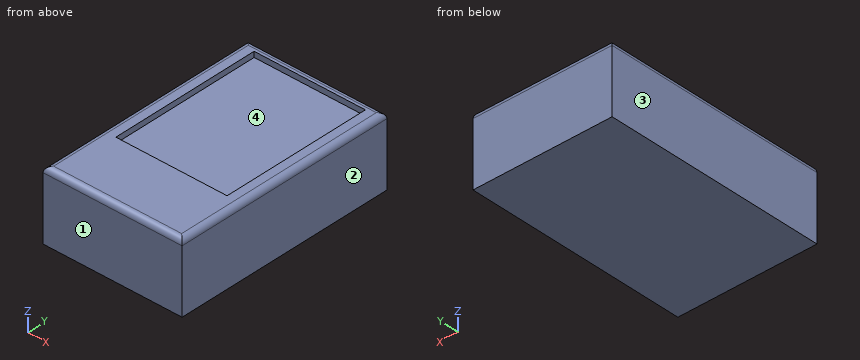
from build123d import *

# Parameters (mm, degrees)
F0_W     = 63.5
F0_H     = 101.6
F1_DEPTH = 31.75
F2_R     = 2.54
F3_W     = 50.8
F3_H     = 68.58
F4_DEPTH = 2.54


with BuildPart() as f1:
    # F0 (on Top) → F1 (new body)
    with BuildSketch(Plane.XY):
        Rectangle(F0_W, F0_H)
    extrude(amount=F1_DEPTH)

    # F2
    f2_edges = [f1.edges().sort_by_distance(p)[0] for p in [
        (0, 50.8, 31.75),
        (-31.75, 0, 31.75),
        (31.75, 0, 31.75),
        (0, -50.8, 31.75),
    ]]
    fillet(f2_edges, radius=F2_R)

    # F3 (on face) → F4 (cut)
    with BuildSketch(Plane.XY.offset(31.75)):
        with Locations((0, 12.7)):
            Rectangle(F3_W, F3_H)
    extrude(amount=-F4_DEPTH, mode=Mode.SUBTRACT)


solid = f1.part
Verification items for the finished model (mm, model axes). Face numbers are marked on the shaded views. Round coordinates to 2 decimals unless told otherwise and drop trailing zeros. Loops run counter-clockwise (first coordinate to the right, second up) from the corner with the lowest first, then second, coordinate; pieces in that order, holes last. Notation, with made-up numbers: M 55,23.25 L 98,23.25 A9 ccw 98,35.25 Z; hole C -19,-24.5 d10. An arc over 180 degrees is marked long. Write each question's results on one line, items separated by ' | '.
1) Section check B-B on y = 11. Record the boundary of the cut face in (x, z).
Checks:
outline: M -31.75,0 L 31.75,0 L 31.75,29.21 A2.54 ccw 29.21,31.75 L 25.4,31.75 L 25.4,29.21 L -25.4,29.21 L -25.4,31.75 L -29.21,31.75 A2.54 ccw -31.75,29.21 Z
2) Gauge pin test, flat ends, axial feed: P1, Ø2, axis at x = 9, z = 30.5, coming from the +Y side; P2, Ø0.8, axis at y = 0, z = 31, coming from the -X side; P3, Ø6, axis at x = -0.5, y = -18, coming from the +Z side. Record the tip position at first contact, or that the pin passes through.
Checks:
P1: stops at y = 50.78 | P2: stops at x = -31.34 | P3: stops at z = 29.21
3) Section check A-A on x = -3.5. Record the boundary of the cut face in (y, z), then the cut area to 3 significant figures.
Checks:
outline: M -50.8,0 L 50.8,0 L 50.8,29.21 A2.54 ccw 48.26,31.75 L 46.99,31.75 L 46.99,29.21 L -21.59,29.21 L -21.59,31.75 L -48.26,31.75 A2.54 ccw -50.8,29.21 Z | area: 3,050 mm2
4) Mould release check, pull along X, two halves, no side actions. Record for the marked faces 1, 2, 3 and 4: released by +X, released by -X, zero draft, split by the parting line, or undercut.
Checks:
face 1: zero draft | face 2: released by +X | face 3: released by -X | face 4: undercut
5) Scan lines: L1, parallel to Z at x = -9, y = -7.5; L2, parallel to Y at x = -4.5, z = 30.5; L3, parallel to X at y = -27, z = 30. Record each from-to range of solid material in increasing order. Write a range as from..to.
Checks:
L1: z = 0..29.21 | L2: y = -50.45..-21.59, 46.99..50.45 | L3: x = -31.62..31.62
